from build123d import *

# Parameters (mm, degrees)
F0_R     = 8.1133177019
F1_DEPTH = 20
F3_DEPTH = 15
F5_DEPTH = 25
F7_DEPTH = 80


# Not quite as in the source:
# - a feature names something its author has since deleted; it is built from what else it names


with BuildPart() as f1:
    # F0 (on Front) → F1 (new body)
    with BuildSketch(Plane.XZ):
        Circle(F0_R)
    extrude(amount=F1_DEPTH)

    # F2 (on Right) → F3 (join)
    with BuildSketch(Plane.YZ):
        Polygon((0, -6.4580785111), (0, 5.4941866547), (-15.2294980362, 3.7591799628), (-15.2294980362, -3.7591799628), align=None)
    extrude(amount=F3_DEPTH)

    # F4 (on Right) → F5 (join)
    with BuildSketch(Plane.YZ):
        with BuildLine():
            ThreePointArc((-4.1447370313, 0), (-2.9307716611, -2.9307716611), (0, -4.1447370313))
            Line((0, -4.1447370313), (0, 4.1447370313))
            ThreePointArc((0, 4.1447370313), (-2.9307716611, 2.9307716611), (-4.1447370313, 0))
        make_face()
    extrude(amount=F5_DEPTH)

    # F6 (on Right) → F7 (join)
    with BuildSketch(Plane.YZ):
        with BuildLine():
            ThreePointArc((-2.6943630073, 0), (-1.9052023535, -1.9052023535), (0, -2.6943630073))
            Line((0, -2.6943630073), (0, 2.6943630073))
            ThreePointArc((0, 2.6943630073), (-1.9052023535, 1.9052023535), (-2.6943630073, 0))
        make_face()
    extrude(amount=F7_DEPTH)


solid = f1.part
CAD build for the part. Positions are in the model's coordinates, mm. A direction names the side the tool comes from. Coordinates: 2 decimals unless noted, no trailing zeros. Write each loop counter-clockwise with the first axis right and the second up, starting at its lowest first coordinate (ties: lowest second). Pieces come first, ordered by that corner, then holes. Notation, with made-up numbers: M 63.25,65.5 L 93.25,65.5 A30 ccw 93.25,96.5 Z; hole C -26,20.25 d7. An arc over 180 degrees is marked long. Return JSON: item names as keys, results as strings.
Item 1: Drop flat-ended pins along their axis: pin 1 Ø8 at (x, y) = (1, -17) entering from -Z; pin 2 Ø2 at (y, z) = (-6, -3.5) entering from +X; pin 3 Ø6 at (x, z) = (64.5, 2) entering from -Y; pin 4 Ø8 at (x, z) = (18.5, 2.5) entering from -Y. Give the stop position or say it passes through.
Findings below:
{"pin 1": "stops at z = -8.11", "pin 2": "stops at x = 15", "pin 3": "stops at y = -2.69", "pin 4": "stops at y = -15.23"}
Item 2: Slice it at C-C, the plane z = 6.5. Write the cut outline in (x, y), and give its area (3 significant figures).
Findings below:
{"outline": "M -4.86,-20 L 4.86,-20 L 4.86,0 L -4.86,0 Z", "area": "194 mm2"}
Item 3: Probe line 1 (X direction, y = -9.5, z = 0.25); line 2 (Y direction, x = 13.5, z = 2.75); line 3 (X direction, y = -1.75, z = 3.25). List the from-to ranges inside material, lowest first. Write a range as from..to.
Findings below:
{"line 1": "x = -8.11..15", "line 2": "y = -15.23..0", "line 3": "x = -7.43..25"}
Item 4: Slice it at B-B, the plane y = -18.25. Write the cut outline in (x, z), and give its area (3 significant figures).
Findings below:
{"outline": "C 0,0 d16.23", "area": "207 mm2"}
Item 5: Which spindle directions (+Z, -Z, +X, -X, +Y, -Y) get a long thin tool onto all of the face, cutting with end or side? Do faces 1 (the flat face through (11.01, -7.72, -5.09)), 2 (the flat face through (25, -3, 0)), 3 (the flat face through (10.42, -7.51, 4.64)), 4 (the flat face through (0, -20, 0)), 5 (the flat face through (26, 0, 0)). Say none if no direction does.
Findings below:
{"face 1": "-Z, +X, -Y", "face 2": "+X, -Y", "face 3": "+Z, +X, -Y", "face 4": "+Z, -Z, +X, -X, -Y", "face 5": "+Z, -Z, +X, -X, +Y"}
Item 6: Slice it at D-D, the plane x = 34. Write the cut outline in (y, z).
Findings below:
{"outline": "M 0,-2.69 L 0,2.69 A2.69 ccw Z"}
Item 7: Slice it at A-A, the plane x = 17.5. Write the cut outline in (y, z), and give its area (3 significant figures).
Findings below:
{"outline": "M 0,-4.14 L 0,4.14 A4.14 ccw Z", "area": "27.0 mm2"}
